```python
from build123d import *

# Parameters (mm, degrees)
SKETCH_1_R          = 2
EXTRUDE_1_DEPTH     = 1
SKETCH_2_R          = 1.5
EXTRUDE_2_DEPTH     = 4
FILLET_1_R          = 1.4
CUT_EXTRUDE_1_DEPTH = 4
SKETCH_4_W          = 0.5
SKETCH_4_H          = 0.5
EXTRUDE_3_DEPTH     = 4


with BuildPart() as part:
    # Эскиз1 → Бобышка-Вытянуть1 (new body)
    with BuildSketch(Plane(origin=(0, 0, 0), x_dir=(1, 0, 0), z_dir=(0, 1, 0))):
        Circle(SKETCH_1_R)
    extrude(amount=EXTRUDE_1_DEPTH)

    # Эскиз2 → Бобышка-Вытянуть2 (add)
    with BuildSketch(Plane(origin=(0, 0, 0), x_dir=(-1, 0, 0), z_dir=(0, -1, 0))):
        Circle(SKETCH_2_R)
    extrude(amount=EXTRUDE_2_DEPTH)

    # Скругление1
    fillet_1_edges = [part.edges().sort_by_distance(p)[0] for p in [
        (1.5, -4, 0),
    ]]
    fillet(fillet_1_edges, radius=FILLET_1_R)

    # Эскиз3 → Вырез-Вытянуть1 (cut)
    with BuildSketch(Plane.XZ):
        with BuildLine():
            Line((-1.322875656, 1.5), (1.322875656, 1.5))
            ThreePointArc((1.322875656, 1.5), (0, 2), (-1.322875656, 1.5))
        make_face()
    extrude(amount=-CUT_EXTRUDE_1_DEPTH, mode=Mode.SUBTRACT)

    # Эскиз4 → Бобышка-Вытянуть3 (add)
    with BuildSketch(Plane(origin=(0, 1, 0), x_dir=(1, 0, 0), z_dir=(0, 1, 0))):
        with Locations((0, -1.103924033)):
            Rectangle(SKETCH_4_W, SKETCH_4_H)
        with Locations((0, 1.575495182)):
            Rectangle(SKETCH_4_W, SKETCH_4_H)
    extrude(amount=EXTRUDE_3_DEPTH)


solid = part.part
```
Could you check a few things on this model? Use its own coordinates, in mm. A direction names the side the tool comes from. Round coordinates to 2 decimals unless told otherwise and drop trailing zeros. Loops run counter-clockwise (first coordinate to the right, second up) from the corner with the lowest first, then second, coordinate; pieces in that order, holes last. Notation, with made-up numbers: (15.25, 51) - (57.25, 51) arc R30 cw to (57.25, 75) - close; hole circle Ø3 at (39, -35). An arc over 180 degrees is marked (long way). Answer as CSV lines item,"result".
1. I want a section at A-A on y = 4. List the corners of the cut face in (x, z) for me, then the cut area to 3 significant figures.
Filled in:
outline,"(-0.25, -1.83) - (0.25, -1.83) - (0.25, -1.33) - (-0.25, -1.33) - close; (-0.25, 0.85) - (0.25, 0.85) - (0.25, 1.35) - (-0.25, 1.35) - close"
area,"0.500 mm^2"
2. Please list where these lines run through material, in increasing order: line 1 along Z through (x, y) = (0.05, 3.75); line 2 along X through (y, z) = (1.75, 1); line 3 along Y through (x, z) = (1.5, 1.2). Write a range as [from, to].
Filled in:
line 1,"z = [-1.83, -1.33], [0.85, 1.35]"
line 2,"x = [-0.25, 0.25]"
line 3,"y = [0, 1]"
3. For pin 1 Ø1 at (x, z) = (-1.5, 1) entering from -Y; pin 2 Ø0.6 at (y, z) = (3.5, -1.5) entering from +X; pin 3 Ø1.8 at (x, z) = (0, -0.5) entering from +Y; pin 4 Ø0.6 at (y, z) = (3, 1) entering from -X, each with a flat end and sliding along its axis, tell me the tip position at first contact or that it passes through.
Filled in:
pin 1,"stops at y = -3.32"
pin 2,"stops at x = 0.25"
pin 3,"stops at y = 5"
pin 4,"stops at x = -0.25"
4. I want a section at B-B on y = -1.5. List the corners of the cut face in (x, z) for me, then the cut area to 3 significant figures.
Filled in:
outline,"circle Ø3 at (0, 0)"
area,"7.07 mm^2"
5. On a 3-axis mill with a long thin cutter (end or side, diameter ignored), from which of +Z, -Z, +X, -X, +Y, -Y can I reach the whole of each face in a straight line? I mean faces 1 (the face through (0, 0.5, 1.5)), 2 (the face through (1.5, -1.28, -0.07)). Say none if no direction works.
Filled in:
face 1,"+Z, +X, -X, +Y, -Y"
face 2,"-Y"
